```python
from build123d import *

# Parameters (mm, degrees)
F1_DEPTH = 25
F2_R     = 1.6101418037
F3_DEPTH = 25
F5_DEPTH = 70
F6_W     = 3.75
F6_H     = 58.5
F7_DEPTH = 30.001
F8_W     = 20
F8_H     = 48.5
F9_DEPTH = 25
F10_R    = 5
F11_R    = 2


with BuildPart() as f1:
    # F0 (on Top) → F1 (new body)
    with BuildSketch(Plane.XY):
        with BuildLine():
            Line((15, 4), (3.9, 4))
            ThreePointArc((3.9, 4), (0, 0.1), (-3.9, 4))
            Line((-3.9, 4), (-15, 4))
            Line((-15, 4), (-15, -4))
            Line((-15, -4), (15, -4))
            Line((15, -4), (15, 4))
        make_face()
    extrude(amount=F1_DEPTH)

    # F2 (on face) → F3 (cut)
    with BuildSketch(Plane.XZ.offset(4)):
        with Locations((-10, 20)):
            Circle(F2_R)
        with Locations((-10, 5)):
            Circle(F2_R)
        with Locations((10, 20)):
            Circle(F2_R)
        with Locations((10, 5)):
            Circle(F2_R)
    extrude(amount=-F3_DEPTH, mode=Mode.SUBTRACT)

    # F4 (on face) → F5 (join)
    with BuildSketch(Plane.XY.offset(25)):
        with BuildLine():
            Line((-15, 4), (-15, -4))
            Line((-15, -4), (15, -4))
            Line((15, -4), (15, 4))
            Line((15, 4), (3.9, 4))
            ThreePointArc((3.9, 4), (0, 0.1), (-3.9, 4))
            Line((-3.9, 4), (-15, 4))
        make_face()
        with BuildLine():
            Line((3.9, 4), (-3.9, 4))
            ThreePointArc((-3.9, 4), (0, 0.1), (3.9, 4))
        make_face()
    extrude(amount=F5_DEPTH)

    # F6 (on face) → F7 (cut, through all)
    with BuildSketch(Plane(origin=(-15, 0, 0), x_dir=(0, -1, 0), z_dir=(-1, 0, 0))):
        with Locations((-2.125, 59.25)):
            Rectangle(F6_W, F6_H)
    extrude(amount=-F7_DEPTH, mode=Mode.SUBTRACT)

    # F8 (on face) → F9 (cut)
    with BuildSketch(Plane(origin=(0, 0.25, 0), x_dir=(-1, 0, 0), z_dir=(0, 1, 0))):
        with Locations((0, 59.25)):
            Rectangle(F8_W, F8_H)
    extrude(amount=-F9_DEPTH, mode=Mode.SUBTRACT)

    # F10
    f10_edges = [f1.edges().sort_by_distance(p)[0] for p in [
        (10, -1.875, 35),
        (-10, -1.875, 83.5),
        (-10, -1.875, 35),
        (10, -1.875, 83.5),
    ]]
    fillet(f10_edges, radius=F10_R)

    # F11
    f11_edges = [f1.edges().sort_by_distance(p)[0] for p in [
        (0, -4, 95),
    ]]
    fillet(f11_edges, radius=F11_R)


solid = f1.part
```
Geometry: final body of the model. Coordinates: model frame, mm. A direction names the side the tool comes from. Round coordinates to 2 decimals unless told otherwise and drop trailing zeros. Loops run counter-clockwise (first coordinate to the right, second up) from the corner with the lowest first, then second, coordinate; pieces in that order, holes last.
Item 1: Contact query for flat-ended pins moving along their axis: P1, Ø4.5, axis at x = 1, y = 3, coming from the -Z side; P2, Ø3.5, axis at x = -10, z = 5, coming from the +Y side; P3, Ø1.5, axis at x = 10, z = 81, coming from the +Y side. Output: stop coordinate, or through.
Checked values:
P1: stops at z = 25
P2: stops at y = 4
P3: stops at y = 0.25
Item 2: Section C-C, the plane y = 2. Output: boundary loops of the cut face in (x, z).
Checked values:
outline: (-15, 0) - (-3.35, 0) - (-3.35, 25) - (3.35, 25) - (3.35, 0) - (15, 0) - (15, 30) - (-15, 30) - close; (-15, 88.5) - (15, 88.5) - (15, 95) - (-15, 95) - close; hole circle Ø3.22 at (-10, 5); hole circle Ø3.22 at (-10, 20); hole circle Ø3.22 at (10, 5); hole circle Ø3.22 at (10, 20)
Item 3: Section B-B, the plane x = 0. Output: boundary loops of the cut face in (y, z).
Checked values:
outline: (-4, 0) - (0.1, 0) - (0.1, 25) - (4, 25) - (4, 30) - (0.25, 30) - (0.25, 35) - (-4, 35) - close; (-4, 83.5) - (0.25, 83.5) - (0.25, 88.5) - (4, 88.5) - (4, 95) - (-2, 95) arc R2 ccw to (-4, 93) - close
Item 4: Mould query, pull axis X, two halves, no side actions, for faces 1 (the flat face through (15, -1, 47)), 2 (the flat face through (0, -2, 83.5)), 3 (the flat face through (0, 1, 95)). Classes: released by +X, released by -X, zero draft, split by the parting line, or undercut.
Checked values:
face 1: released by +X
face 2: undercut
face 3: zero draft
Item 5: Reachability of faces 4 (the flat face through (0, 3, 25)), 5 (the flat face through (0, 2, 88.5)), 6 (the cylindrical face through (8.57, -1.9, 82)) from +Z, -Z, +X, -X, +Y, -Y: full face, straight path, thin tool, end or side. Return the list, or none.
Checked values:
face 4: -Z, +Y
face 5: +X, -X, +Y
face 6: +Y, -Y
Item 6: Section A-A, the plane z = 71. Output: boundary loops of the cut face in (x, y).
Checked values:
outline: (-15, -4) - (-10, -4) - (-10, 0.25) - (-15, 0.25) - close; (10, -4) - (15, -4) - (15, 0.25) - (10, 0.25) - close
Item 7: Section D-D, the plane z = 5. Output: boundary loops of the cut face in (x, y).
Checked values:
outline: (-15, -4) - (-11.61, -4) - (-11.61, 4) - (-15, 4) - close; (-8.39, -4) - (8.39, -4) - (8.39, 4) - (3.9, 4) arc R3.9 cw to (-3.9, 4) - (-8.39, 4) - close; (11.61, -4) - (15, -4) - (15, 4) - (11.61, 4) - close
Item 8: Line query: L1, parallel to Z at x = -10, y = 2; L2, parallel to X at y = -0.25, z = 73.5; L3, parallel to Z at x = -1.75, y = -1. Output: solid intervals per line, ascending.
Checked values:
L1: z = 0 to 3.39, 6.61 to 18.39, 21.61 to 30, 88.5 to 95
L2: x = -15 to -10, 10 to 15
L3: z = 0 to 35, 83.5 to 95
